Read the model definition and answer for the solid it produces. Units are mm, in the model's axes. Face numbers are marked on the shaded views. A direction names the side the tool comes from. Coordinates: 2 decimals unless noted, no trailing zeros. Write each loop counter-clockwise with the first axis right and the second up, starting at its lowest first coordinate (ties: lowest second). Pieces come first, ordered by that corner, then holes.
(1) Straight lines are drawn through the part: line 1 along X through (y, z) = (4.5, -11.56) (3 decimals); line 2 along X through (y, z) = (13.5, 14) (3 decimals); line 3 along Z through (x, y) = (38, 9.5). For each, find the intervals that lie inside material, in ascending order.
(2) The part is cut by section A-A, the plane z = -11.56. Determine the outline of the cut face in (x, y) (3 decimals).
(3) The part is cut by section D-D, the plane z = 40.5. Determine the outline of the cut face in (x, y) (3 decimals), and give its area (3 significant figures).
(4) The part is cut by section B-B, the plane y = 6. State how many separate pieces and enclosed holes the cut face has, and give its area (3 significant figures).
(5) The part is cut by section C-C, the plane x = 15.5. Determine the outline of the cut face in (y, z).
(6) Given pin 1 (3 mm diameter, centred on y = 5, z = 8, fed in from +X); pin 2 (8 mm diameter, centred on x = 58.5, z = 6, fed in from +Y); pin 3 (4 mm diameter, centred on x = 36.325, z = 28.44, fed in from -Y); pin 4 (2 mm diameter, centred on y = 15, z = -40, fed in from +X), each flat-ended and moving along its own axis, determine where each tip first touches the part or whether it passes through.
(7) Which of the six approach directions +Z, -Z, +X, -X, +Y, -Y give full straight-line access (tool end or side, diameter ignored) to the marked faces 1, 2 and 3?
```python
from build123d import *

# Parameters (mm, degrees)
BOSS_EXTRUDE1_DEPTH            = 112.65
M4X0_7_TAPPED_HOLE1_AT_2_COUNT = 2
M4X0_7_TAPPED_HOLE1_AT_2_PITCH = 50
M4X0_7_TAPPED_HOLE1_AT_3_COUNT = 2
M4X0_7_TAPPED_HOLE1_AT_3_PITCH = 52.201532545
SKETCH7_W                      = 10
SKETCH7_H                      = 54.452673799
CUT_EXTRUDE2_DEPTH             = 80
CSK_FOR_M4_SFHCS1_AT_2_COUNT   = 2
CSK_FOR_M4_SFHCS1_AT_2_PITCH   = 40
CSK_FOR_M4_SFHCS1_AT_3_COUNT   = 2
CSK_FOR_M4_SFHCS1_AT_3_PITCH   = 27.92
CSK_FOR_M4_SFHCS1_AT_4_COUNT   = 2
CSK_FOR_M4_SFHCS1_AT_4_PITCH   = 12.08
SKETCH11_W                     = 12
SKETCH11_H                     = 10
CUT_EXTRUDE3_DEPTH             = 156.060918939
FILLET1_R                      = 15


with BuildPart() as part:
    # Sketch1 → Boss-Extrude1 (new body)
    with BuildSketch(Plane(origin=(0, 0, 0), x_dir=(0, 0, -1), z_dir=(1, 0, 0))):
        Polygon((-50, 10), (-50, 0), (50, 0), (50, 36.794919243), align=None)
    extrude(amount=BOSS_EXTRUDE1_DEPTH)

    # Sketch5 → M4x0.7 Tapped Hole1 (revolve, cut)
    with BuildSketch(Plane(origin=(112.65, 15, 10), x_dir=(0, 0, -1), z_dir=(0, 1, 0))):
        Polygon((0, 0), (0, 11.091420021), (1.65, 10.1), (1.65, 0), align=None)
    m4x0_7_tapped_hole1 = revolve(axis=Axis((119, 15, 10), (-1, 0, 0)), mode=Mode.SUBTRACT)

    # M4x0.7 Tapped Hole1 at 2: M4x0.7 Tapped Hole1 ×2
    with Locations(*[(0, 0, -i * M4X0_7_TAPPED_HOLE1_AT_2_PITCH) for i in range(1, M4X0_7_TAPPED_HOLE1_AT_2_COUNT)]):
        add(m4x0_7_tapped_hole1, mode=Mode.SUBTRACT)

    # M4x0.7 Tapped Hole1 at 3: M4x0.7 Tapped Hole1 ×2
    with Locations(*[Vector(0, 0.28734788556634544, -0.9578262852211514) * (i * M4X0_7_TAPPED_HOLE1_AT_3_PITCH) for i in range(1, M4X0_7_TAPPED_HOLE1_AT_3_COUNT)]):
        add(m4x0_7_tapped_hole1, mode=Mode.SUBTRACT)

    # Sketch7 → Cut-Extrude2 (cut)
    with BuildSketch(Plane.XY.offset(50)):
        with Locations((76.325, 37.2263369)):
            Rectangle(SKETCH7_W, SKETCH7_H)
    cut_extrude2 = extrude(amount=-CUT_EXTRUDE2_DEPTH, mode=Mode.SUBTRACT)

    # Sketch10 → CSK for M4 SFHCS1 (revolve, cut)
    with BuildSketch(Plane(origin=(76.325, 10, -11.56), x_dir=(0, 0, 1), z_dir=(1, 0, 0))):
        Polygon((0, 0), (0, 11.451936393), (2.25, 10.1), (2.25, 2.23), (4.48, 0), align=None)
    csk_for_m4_sfhcs1 = revolve(axis=Axis((76.325, 16.35, -11.56), (0, -1, 0)), mode=Mode.SUBTRACT)

    # CSK for M4 SFHCS1 at 2: CSK for M4 SFHCS1 ×2
    with Locations(*[(0, 0, i * CSK_FOR_M4_SFHCS1_AT_2_PITCH) for i in range(1, CSK_FOR_M4_SFHCS1_AT_2_COUNT)]):
        add(csk_for_m4_sfhcs1, mode=Mode.SUBTRACT)

    # CSK for M4 SFHCS1 at 3: CSK for M4 SFHCS1 ×2
    with Locations(*[(0, 0, i * CSK_FOR_M4_SFHCS1_AT_3_PITCH) for i in range(1, CSK_FOR_M4_SFHCS1_AT_3_COUNT)]):
        add(csk_for_m4_sfhcs1, mode=Mode.SUBTRACT)

    # CSK for M4 SFHCS1 at 4: CSK for M4 SFHCS1 ×2
    with Locations(*[(0, 0, -i * CSK_FOR_M4_SFHCS1_AT_4_PITCH) for i in range(1, CSK_FOR_M4_SFHCS1_AT_4_COUNT)]):
        add(csk_for_m4_sfhcs1, mode=Mode.SUBTRACT)

    # Sketch11 → Cut-Extrude3 (cut, through all)
    with BuildSketch(Plane.XY.offset(50)):
        with Locations((106.65, 5)):
            Rectangle(SKETCH11_W, SKETCH11_H)
    cut_extrude3 = extrude(amount=-CUT_EXTRUDE3_DEPTH, mode=Mode.SUBTRACT)

    # Mirror1: M4x0.7 Tapped Hole1, Cut-Extrude2, CSK for M4 SFHCS1, Cut-Extrude3 across plane
    add(m4x0_7_tapped_hole1.mirror(Plane.ZY.offset(-56.325)), mode=Mode.SUBTRACT)
    add(cut_extrude2.mirror(Plane.ZY.offset(-56.325)), mode=Mode.SUBTRACT)
    add(csk_for_m4_sfhcs1.mirror(Plane.ZY.offset(-56.325)), mode=Mode.SUBTRACT)
    add(cut_extrude3.mirror(Plane.ZY.offset(-56.325)), mode=Mode.SUBTRACT)

    # Mirror1 copy 1 sketch → Mirror1 copy 1 (revolve, cut)
    with BuildSketch(Plane(origin=(0, 15, -40), x_dir=(0, 0, -1), z_dir=(0, 1, 0))):
        Polygon((0, 0), (0, -11.091420021), (1.65, -10.1), (1.65, 0), align=None)
    revolve(axis=Axis((-6.35, 15, -40), (-1, 0, 0)), mode=Mode.SUBTRACT)

    # Mirror1 copy 2 sketch → Mirror1 copy 2 (revolve, cut)
    with BuildSketch(Plane(origin=(0, 30, -40), x_dir=(0, 0, -1), z_dir=(0, 1, 0))):
        Polygon((0, 0), (0, -11.091420021), (1.65, -10.1), (1.65, 0), align=None)
    revolve(axis=Axis((-6.35, 30, -40), (-1, 0, 0)), mode=Mode.SUBTRACT)

    # Mirror1 copy 3 sketch → Mirror1 copy 3 (revolve, cut)
    with BuildSketch(Plane(origin=(36.325, 10, 28.44), x_dir=(0, 0, 1), z_dir=(-1, 0, 0))):
        Polygon((0, 0), (0, -11.451936393), (2.25, -10.1), (2.25, -2.23), (4.48, 0), align=None)
    revolve(axis=Axis((36.325, 16.35, 28.44), (0, 1, 0)), mode=Mode.SUBTRACT)

    # Mirror1 copy 4 sketch → Mirror1 copy 4 (revolve, cut)
    with BuildSketch(Plane(origin=(36.325, 10, 16.36), x_dir=(0, 0, 1), z_dir=(-1, 0, 0))):
        Polygon((0, 0), (0, -11.451936393), (2.25, -10.1), (2.25, -2.23), (4.48, 0), align=None)
    revolve(axis=Axis((36.325, 16.35, 16.36), (0, 1, 0)), mode=Mode.SUBTRACT)

    # Mirror1 copy 5 sketch → Mirror1 copy 5 (revolve, cut)
    with BuildSketch(Plane(origin=(36.325, 10, -23.64), x_dir=(0, 0, 1), z_dir=(-1, 0, 0))):
        Polygon((0, 0), (0, -11.451936393), (2.25, -10.1), (2.25, -2.23), (4.48, 0), align=None)
    revolve(axis=Axis((36.325, 16.35, -23.64), (0, 1, 0)), mode=Mode.SUBTRACT)

    # Fillet1
    fillet1_edges = [part.edges().sort_by_distance(p)[0] for p in [
        (12, 5, 50),
        (12, 5, -50),
        (100.65, 5, -50),
        (100.65, 5, 50),
    ]]
    fillet(fillet1_edges, radius=FILLET1_R)


solid = part.part
```
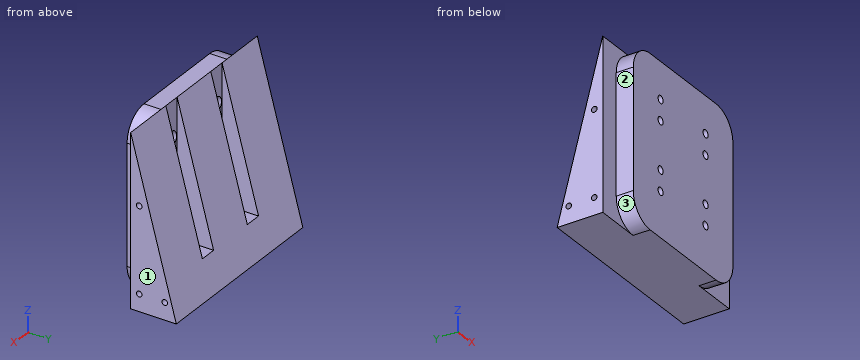
Computed:
1. line 1: x = 12 to 34.075, 38.575 to 74.075, 78.575 to 100.65
1. line 2: x = 0 to 31.325, 41.325 to 71.325, 81.325 to 112.65
1. line 3: z = -50 to -27.25, -20.03 to -15.17, -7.95 to 12.75, 19.97 to 24.83, 32.05 to 50
2. outline: (0, 10) - (12, 10) - (12, 0) - (34.075, 0) - (34.075, 7.77) - (31.845, 10) - (31.325, 10) - (31.325, 26.495) - (0, 26.495) - close; (38.575, 0) - (74.075, 0) - (74.075, 7.77) - (71.845, 10) - (71.325, 10) - (71.325, 26.495) - (41.325, 26.495) - (41.325, 10) - (40.805, 10) - (38.575, 7.77) - close; (78.575, 0) - (100.65, 0) - (100.65, 10) - (112.65, 10) - (112.65, 26.495) - (81.325, 26.495) - (81.325, 10) - (80.805, 10) - (78.575, 7.77) - close
3. outline: (0, 10) - (13.045, 10) - (13.045, 0) - (99.605, 0) - (99.605, 10) - (112.65, 10) - (112.65, 12.546) - (81.325, 12.546) - (81.325, 10) - (71.325, 10) - (71.325, 12.546) - (41.325, 12.546) - (41.325, 10) - (31.325, 10) - (31.325, 12.546) - (0, 12.546) - close
3. area: 1,100 mm2
4. separate pieces: 1
4. enclosed holes: 8
4. area: 8,540 mm2
5. outline: (0, -44.63) - (10, -44.63) - (10, -50) - (36.79, -50) - (10, 50) - (10, 44.63) - (0, 44.63) - close
6. pin 1: stops at x = 100.65
6. pin 2: stops at y = 22.86
6. pin 3: passes through
6. pin 4: stops at x = 102.16
7. face 1: +Z, -Z, +X, +Y, -Y
7. face 2: +Z, -Z, -X, -Y
7. face 3: -Z, -X, -Y
